from build123d import *

# Parameters (mm, degrees)
SKETCH_1_W               = 20
SKETCH_1_H               = 100
EXTRUDE_1_DEPTH          = 3
SKETCH_2_R               = 1.5
CUT_EXTRUDE_1_DEPTH      = 52.078371156
CUT_EXTRUDE_2_DEPTH      = 52.078371156
CUT_EXTRUDE_2_DEPTH_BACK = 52.078371156
SKETCH_3_W               = 5
SKETCH_3_H               = 60
FILLET_1_R               = 3
FILLET_2_R               = 3
SKETCH_4_R               = 1.5
CUT_EXTRUDE_3_DEPTH      = 52.078371156


with BuildPart() as part:
    # 草图1 → 凸台-拉伸1 (new body)
    with BuildSketch(Plane(origin=(0, 0, 0), x_dir=(1, 0, 0), z_dir=(0, 1, 0))):
        Rectangle(SKETCH_1_W, SKETCH_1_H)
    extrude(amount=EXTRUDE_1_DEPTH)

    # 草图2 → 切除-拉伸1 (cut, through all)
    with BuildSketch(Plane(origin=(0, 3, 0), x_dir=(1, 0, 0), z_dir=(0, 1, 0))):
        with Locations(Location((-7.5, 45, 0), (0, 0, 270))):
            Circle(SKETCH_2_R)
        with Locations(Location((-7.5, 35, 0), (0, 0, 270))):
            Circle(SKETCH_2_R)
        with Locations(Location((7.5, 45, 0), (0, 0, 90))):
            Circle(SKETCH_2_R)
        with Locations(Location((7.5, 35, 0), (0, 0, 90))):
            Circle(SKETCH_2_R)
        with Locations(Location((7.5, -35, 0), (0, 0, 270))):
            Circle(SKETCH_2_R)
        with Locations(Location((7.5, -45, 0), (0, 0, 270))):
            Circle(SKETCH_2_R)
        with Locations(Location((-7.5, -35, 0), (0, 0, 90))):
            Circle(SKETCH_2_R)
        with Locations(Location((-7.5, -45, 0), (0, 0, 90))):
            Circle(SKETCH_2_R)
    extrude(amount=-CUT_EXTRUDE_1_DEPTH, mode=Mode.SUBTRACT)

    # 草图3 → 切除-拉伸2 (cut, two sides: drawn at the far end of the back side and taken through both)
    with BuildSketch(Plane(origin=(0, 3, 0), x_dir=(1, 0, 0), z_dir=(0, 1, 0)).offset(-CUT_EXTRUDE_2_DEPTH_BACK)):
        Rectangle(SKETCH_3_W, SKETCH_3_H)
    extrude(amount=CUT_EXTRUDE_2_DEPTH + CUT_EXTRUDE_2_DEPTH_BACK, mode=Mode.SUBTRACT)

    # 圆角1
    # the kernel refuses this fillet: 3 mm, written as the material it adds along each edge
    with BuildSketch(Plane(origin=(-2.5, 3, -30), x_dir=(1, 0, 0), z_dir=(0, -1, 0)), Plane(origin=(-2.5, 3, 30), x_dir=(0, 0, -1), z_dir=(0, -1, 0)), Plane(origin=(2.5, 0, 30), x_dir=(0, 0, -1), z_dir=(0, 1, 0))) as fillet_1_piece_1:
        with BuildLine():
            CenterArc((FILLET_1_R, FILLET_1_R), FILLET_1_R, 180, 90)
            Line((0, FILLET_1_R), (0, 0))
            Line((0, 0), (FILLET_1_R, 0))
        make_face()
    extrude(amount=3)
    with BuildSketch(Plane(origin=(2.5, 0, -30), x_dir=(0, 0, 1), z_dir=(0, 1, 0))) as fillet_1_piece_2:
        with BuildLine():
            CenterArc((FILLET_1_R, -FILLET_1_R), FILLET_1_R, 90, 90)
            Line((0, -FILLET_1_R), (0, 0))
            Line((0, 0), (FILLET_1_R, 0))
        make_face()
    extrude(amount=3)

    # 圆角2
    fillet_2_edges = [part.edges().sort_by_distance(p)[0] for p in [
        (10, 1.5, 50),
        (-10, 1.5, 50),
        (-10, 1.5, -50),
        (10, 1.5, -50),
    ]]
    fillet(fillet_2_edges, radius=FILLET_2_R)

    # 草图4 → 切除-拉伸3 (cut, through all)
    with BuildSketch(Plane(origin=(0, 3, 0), x_dir=(1, 0, 0), z_dir=(0, 1, 0))):
        with Locations(Location((-6, 7, 0), (0, 0, 270))):
            Circle(SKETCH_4_R)
        with Locations(Location((6, 7, 0), (0, 0, 90))):
            Circle(SKETCH_4_R)
        with Locations(Location((6, -7, 0), (0, 0, 270))):
            Circle(SKETCH_4_R)
        with Locations(Location((-6, -7, 0), (0, 0, 90))):
            Circle(SKETCH_4_R)
    extrude(amount=-CUT_EXTRUDE_3_DEPTH, mode=Mode.SUBTRACT)


solid = part.part
Build history of the part. All positions in model axes, mm. A direction names the side the tool comes from. Give positions to 0.01 mm unless a question says otherwise; leave off trailing zeros. Order: outer loops, then holes, each group sorted by start corner. A loop starts at its lowest first (then second) coordinate and runs counter-clockwise, first axis right, second up. Notation, with made-up numbers: M -7,48 L 11,48 A28 cw 11,66 Z; hole C 77,46 d7. An arc over 180 degrees is marked long. Put each result on its own line as item: value.
Item 1: Cut at C-C on y = 1.3. Count the separate pieces of the cut face and the enclosed holes in it, then the cut area to 3 significant figures.
Results are:
separate pieces: 1
enclosed holes: 13
area: 1,620 mm2
Item 2: Cut at D-D on z = 45. Write the cut outline in (x, y).
Results are:
outline: M -10,0 L -9,0 L -9,3 L -10,3 Z; M -6,0 L 6,0 L 6,3 L -6,3 Z; M 9,0 L 10,0 L 10,3 L 9,3 Z
Item 3: Wall check: probe 1 along X at (y, z) = (1.3, -35); probe 2 along Z at (x, y) = (5, 2.15); probe 3 along X at (y, z) = (1, -17). Give the ranges that are in metal, low to high.
Results are:
probe 1: -10 to -9, -6 to 6, 9 to 10
probe 2: -50 to -8.12, -5.88 to 5.88, 8.12 to 50
probe 3: -10 to -2.5, 2.5 to 10
Item 4: Cut at A-A on z = -23.5. Write the cut outline in (x, y).
Results are:
outline: M -10,0 L -2.5,0 L -2.5,3 L -10,3 Z; M 2.5,0 L 10,0 L 10,3 L 2.5,3 Z
Item 5: Which spindle directions (+Z, -Z, +X, -X, +Y, -Y) get a long thin tool onto all of the face, cutting with end or side? Do faces 5 (the face through (-1.77, 1.52, 28.96)), 6 (the face through (-9.14, 1.52, -49.1)). Say none if no direction does.
Results are:
face 5: +Y, -Y
face 6: -Z, -X, +Y, -Y
Item 6: Pull direction Z, two halves, no side cores. Call faces 1 (the face through (-6.6, 1.5, 46.2)), 2 (the face through (9.1, 1.52, -49.14)), 3 (the face through (9.1, 1.52, 49.14)), 4 (the face through (6.07, 1.52, 5.5)): +Z half, -Z half, draft (parallel to the pull), parting line (faces both ways), or undercut.
Results are:
face 1: undercut
face 2: -Z half
face 3: +Z half
face 4: undercut
Item 7: Cut at B-B on z = -7. Write the cut outline in (x, y).
Results are:
outline: M -10,0 L -7.5,0 L -7.5,3 L -10,3 Z; M -4.5,0 L -2.5,0 L -2.5,3 L -4.5,3 Z; M 2.5,0 L 4.5,0 L 4.5,3 L 2.5,3 Z; M 7.5,0 L 10,0 L 10,3 L 7.5,3 Z
